Model file for the job. Use its own axes, mm. Face numbers are marked on the shaded views. A direction names the side the tool comes from. Round coordinates to 2 decimals unless told otherwise and drop trailing zeros. Order: outer loops, then holes, each group sorted by start corner. A loop starts at its lowest first (then second) coordinate and runs counter-clockwise, first axis right, second up. Notation, with made-up numbers: (34.5, -26.75) - (73.5, -26.75) arc R34 cw to (73.5, 4.25) - close; hole circle Ø5 at (-33, -29). An arc over 180 degrees is marked (long way). Put each result on its own line as item: value. Start each with the question number.
Item 1: Saw through at B-B on z = -182. List the corners of the cut face in (x, y), plus the area to 3 significant figures.
Item 2: Mould opens along X. For the marked faces 4, 5 and 6 say: pulls with the +X half, pulls with the -X half, needs draft (parallel to the pull), parting line crosses it, or undercut.
Item 3: Probe probe 1 along X at (y, z) = (17.5, -300); probe 2 along X at (y, z) = (-10, 0); probe 3 along Z at (x, y) = (6, 15). List the from-to ranges inside material, lowest first.
Item 4: Which spindle directions (+Z, -Z, +X, -X, +Y, -Y) get a long thin tool onto all of the face, cutting with end or side? Do the marked faces 1, 2 and 3. Say none if no direction does.
Item 5: Saw through at A-A on y = -17. List the corners of the cut face in (x, z), plus the area to 3 significant figures.
Item 6: Saw through at D-D on z = -80. List the corners of the cut face in (x, y), plus the area to 3 significant figures.
Item 7: Pin check, flat tips, straight feed: pin 1 Ø12 at (y, z) = (-20, -309.5) entering from -X; pin 2 Ø10 at (x, y) = (37, 5.5) entering from -Z; pin 3 Ø10 at (y, z) = (-13.5, -39.5) entering from +X. Stop position of each tip, or through.
Item 8: Saw through at C-C on x = 0. State how many separate pieces and enclosed holes the cut face has, plus the area to 3 significant figures.
```python
from build123d import *

# Parameters (mm, degrees)
SKETCH1_R             = 45
SKETCH1_R_2           = 22.5
BOSS_EXTRUDE1_DEPTH   = 31.65
SKETCH1_R_3           = 56.25
SKETCH1_R_4           = 28.15
BOSS_EXTRUDE1_2_DEPTH = 31.65
BOSS_EXTRUDE2_DEPTH   = 12.5
CUT_EXTRUDE1_DEPTH    = 5
CUT_EXTRUDE2_START    = -5
CUT_EXTRUDE2_DEPTH    = 5
FILLET1_R             = 5


with BuildPart() as part:
    # Sketch1 → Boss-Extrude1 (new, symmetric)
    with BuildSketch(Plane(origin=(0, 0, 0), x_dir=(1, 0, 0), z_dir=(0, 1, 0))):
        with Locations(Location((0, 0, 0), (0, 0, 270))):
            Circle(SKETCH1_R)
        with Locations(Location((0, 0, 0), (0, 0, 270))):
            Circle(SKETCH1_R_2, mode=Mode.SUBTRACT)
    extrude(amount=BOSS_EXTRUDE1_DEPTH, both=True)



with BuildPart() as body_2:
    # Sketch1 → Boss-Extrude1 2 (new, symmetric)
    with BuildSketch(Plane(origin=(0, 0, 0), x_dir=(1, 0, 0), z_dir=(0, 1, 0))):
        with Locations(Location((0, 300, 0), (0, 0, 270))):
            Circle(SKETCH1_R_3)
        with Locations(Location((0, 300, 0), (0, 0, 270))):
            Circle(SKETCH1_R_4, mode=Mode.SUBTRACT)
    extrude(amount=BOSS_EXTRUDE1_2_DEPTH, both=True)


with BuildPart() as part_1:
    add(part.part)

    add(body_2.part)  # Boss-Extrude2 merges body 2
    # Sketch2 → Boss-Extrude2 (add, symmetric)
    with BuildSketch(Plane(origin=(0, 0, 0), x_dir=(1, 0, 0), z_dir=(0, 1, 0))):
        with BuildLine():
            Line((-56.210435304, 297.890625), (-44.968348244, -1.6875))
            ThreePointArc((-44.968348244, -1.6875), (0, 45), (44.968348244, -1.6875))
            Line((44.968348244, -1.6875), (56.210435304, 297.890625))
            ThreePointArc((56.210435304, 297.890625), (0, 243.75), (-56.210435304, 297.890625))
        make_face()
    extrude(amount=BOSS_EXTRUDE2_DEPTH, both=True)

    # Sketch3 → Cut-Extrude1 (cut)
    with BuildSketch(Plane(origin=(0, 12.5, 0), x_dir=(1, 0, 0), z_dir=(0, 1, 0))):
        with BuildLine():
            Line((-28.619814412, 229.324907336), (-22.255863805, 59.73892388))
            ThreePointArc((-22.255863805, 59.73892388), (0, 63.75), (22.255863805, 59.73892388))
            Line((22.255863805, 59.73892388), (28.619814412, 229.324907336))
            ThreePointArc((28.619814412, 229.324907336), (0, 223.75), (-28.619814412, 229.324907336))
        make_face()
    extrude(amount=-CUT_EXTRUDE1_DEPTH, mode=Mode.SUBTRACT)

    # Sketch4 → Cut-Extrude2 (cut)
    with BuildSketch(Plane.XZ.offset(12.5).offset(CUT_EXTRUDE2_START)):
        with BuildLine():
            Line((22.255863805, -59.73892388), (28.619814412, -229.324907336))
            ThreePointArc((28.619814412, -229.324907336), (0, -223.75), (-28.619814412, -229.324907336))
            Line((-28.619814412, -229.324907336), (-22.255863805, -59.73892388))
            ThreePointArc((-22.255863805, -59.73892388), (0, -63.75), (22.255863805, -59.73892388))
        make_face()
    extrude(amount=CUT_EXTRUDE2_DEPTH, mode=Mode.SUBTRACT)

    # Fillet1
    fillet1_edges = [part_1.edges().sort_by_distance(p)[0] for p in [
        (0, -31.65, -45),
        (0, 31.65, -356.25),
        (0, -31.65, -356.25),
        (0, 31.65, -45),
    ]]
    fillet(fillet1_edges, radius=FILLET1_R)


solid = part_1.part
```
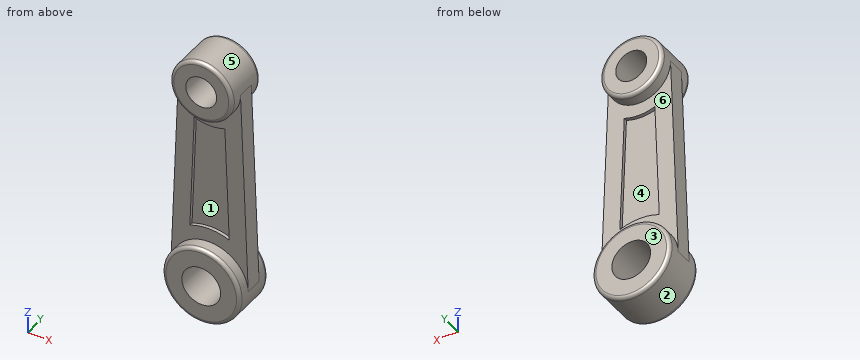
Results found:
1. outline: (-51.86, -12.5) - (-26.84, -12.5) - (-26.84, -7.5) - (26.84, -7.5) - (26.84, -12.5) - (51.86, -12.5) - (51.86, 12.5) - (26.84, 12.5) - (26.84, 7.5) - (-26.84, 7.5) - (-26.84, 12.5) - (-51.86, 12.5) - close
1. area: 2,060 mm²
2. face 4: undercut
2. face 5: parting line crosses it
2. face 6: needs draft
3. probe 1: x = -56.25 to -28.15, 28.15 to 56.25
3. probe 2: x = -45.03 to -22.5, 22.5 to 45.03
3. probe 3: z = -355.93 to -327.5, -272.5 to -244.07, -44.6 to -21.69, 21.69 to 44.6
4. face 1: -Y
4. face 2: none
4. face 3: +Z, -Z, +X, -X, +Y
5. outline: circle Ø112.5 at (0, -300); circle Ø90 at (0, 0); hole circle Ø56.3 at (0, -300); hole circle Ø45 at (0, 0)
5. area: 12,200 mm²
6. outline: (-48.03, -12.5) - (-23.02, -12.5) - (-23.02, -7.5) - (23.02, -7.5) - (23.02, -12.5) - (48.03, -12.5) - (48.03, 12.5) - (23.02, 12.5) - (23.02, 7.5) - (-23.02, 7.5) - (-23.02, 12.5) - (-48.03, 12.5) - close
6. area: 1,940 mm²
7. pin 1: stops at x = -56.14
7. pin 2: stops at z = -346.26
7. pin 3: stops at x = 46.7
8. separate pieces: 3
8. enclosed holes: 0
8. area: 9,730 mm²
